Autodesk Inventor part; units mm, degrees
ref_plane "YZ Plane" through (0, 0, 0) normal (1, 0, 0) x (0, 1, 0)
ref_plane "XZ Plane" through (0, 0, 0) normal (0, 1, 0) x (-1, 0, 0)
ref_plane "XY Plane" through (0, 0, 0) normal (0, 0, 1) x (1, 0, 0)
sketch "Skizze1" plane through (0, 0, 0) normal (0, 0, 1) x (1, 0, 0)
  circle A0 centre (0, 0) radius 7.45
  line L0 (-0.9, 9) -> (0.9, 9)
  line L1 (0.9, 9) -> (0.9, -9)
  line L2 (0.9, -9) -> (-0.9, -9)
  line L3 (-0.9, -9) -> (-0.9, 9)
  line L4 (-0.9, 9) -> (0.9, -9) construction
  line L5 (0.9, 9) -> (-0.9, -9) construction
  circle A1 centre (0, 0) radius 2.25
  point P0 (-0.9, -2.0622)
  point P1 (0.9, -2.0622)
  point P2 (0.9, -7.3954)
  point P3 (-0.9, -7.3954)
  dimension "d0" = 14.9
  dimension "d1" = 1.8
  dimension "d2" = 4.5
extrude "Extrusion1" add sketch "Skizze1" along normal blind 3 contours A0 L1 A1 | L1 A1 L3 A0 | L3 A1 A0 picked at (0.4002, 5.6965)
sketch "Skizze2" plane through (0, 0, 3) normal (0, 0, 1) x (1, 0, 0)
  line L0 (0.9, -2.0622) -> (0.9, -7.3954)
  arc A0 (0.9, -7.3954) -> (-0.9, -7.3954) centre (0, 0) ccw
  line L1 (-0.9, -7.3954) -> (-0.9, -2.0622)
  arc A1 (0.9, -2.0622) -> (-0.9, -2.0622) centre (0, 0) ccw
  circle A2 centre (0, 0) radius 10
  line L2 (-0.9, 11.3464) -> (0.9, 11.3464)
  line L3 (0.9, 11.3464) -> (0.9, -11.3464)
  line L4 (0.9, -11.3464) -> (-0.9, -11.3464)
  line L5 (-0.9, -11.3464) -> (-0.9, 11.3464)
  line L6 (-0.9, 11.3464) -> (0.9, -11.3464) construction
  line L7 (0.9, 11.3464) -> (-0.9, -11.3464) construction
  point P0 (-0.9, -9.9594)
  point P1 (-0.9, 2.0622)
  point P2 (-0.9, 7.3954)
  point P3 (0.9, 7.3954)
  point P4 (0.9, 2.0622)
  point P5 (0.9, -9.9594)
  dimension "d5" = 20
  dimension "d6" = 1.8
extrude "Extrusion2" add sketch "Skizze2" along normal blind 0.8 contours A1 L3 A0 L0 | A0 L3 A2 | A1 L5 A0 L3 | A0 L5 A2 L3 | A1 L1 A0 L5 | A0 L5 A2
sketch "Skizze3" plane through (0, 0, 0) normal (0, 0, -1) x (-1, 0, 0)
  line L0 (-0.9, -2.0622) -> (-0.9, -7.3954)
  arc A0 (0.9, -2.0622) -> (-0.9, -2.0622) centre (0, 0) ccw
  line L1 (0.9, -7.3954) -> (0.9, -2.0622)
  arc A1 (0.9, -7.3954) -> (-0.9, -7.3954) centre (0, 0) ccw
  circle A2 centre (0, 0) radius 7.75
  line L2 (0.9, 14.7103) -> (-0.9, 14.7103)
  line L3 (-0.9, 14.7103) -> (-0.9, -14.7103)
  line L4 (-0.9, -14.7103) -> (0.9, -14.7103)
  line L5 (0.9, -14.7103) -> (0.9, 14.7103)
  line L6 (0.9, 14.7103) -> (-0.9, -14.7103) construction
  line L7 (-0.9, 14.7103) -> (0.9, -14.7103) construction
  point P0 (-0.9, -7.6976)
  point P1 (0.9, -7.6976)
  dimension "d9" = 15.5
  dimension "d10" = 1.8
extrude "Extrusion3" add sketch "Skizze3" along normal blind 1.4 contours L0 A1 L3 A0 | L3 A2 A1 | L3 A1 L5 A0 | L3 A2 L5 A1 | L5 A1 L1 A0 | L5 A2 A1
sketch "Skizze4" plane through (0, 0, 3.8) normal (0, 0, 1) x (1, 0, 0)
  circle A0 centre (0, 0) radius 3
extrude "Extrusion4" cut sketch "Skizze4" against normal through all
chamfer "Fase2" distance 0.3 angle 45 1 edges at (0, 7.75, 0)
fillet "Rundung5" radius 6 1 edges at (0, 3, -1.4)
chamfer "Fase3" distance 0.7 angle 45 1 edges at (0, 7.75, -1.4)
fillet "Rundung6" radius 0.5 1 edges at (0, 7.0754, -1.2194)
fillet "Rundung7" radius 0.2 1 edges at (0, 7.75, -0.7)
fillet "Rundung8" radius 0.5 1 edges at (0, 3, 3.8)
properties part number "Buttomplate_BedholePlug"
Geometry: final body of the model. Coordinates: model frame, mm. Give positions to 0.01 mm unless a question says otherwise; leave off trailing zeros. Order: outer loops, then holes, each group sorted by start corner. A loop starts at its lowest first (then second) coordinate and runs counter-clockwise, first axis right, second up. Notation, with made-up numbers: (22.25, 75.25) -> (46.25, 75.25) arc R27 cw to (46.25, 101.25) -> close; hole circle Ø5 at (40, 73.25). An arc over 180 degrees is marked (long way). Write each question's results on one line, items separated by ' | '. Start each with the question number.
1) First-contact query: pin 1 (2 mm diameter, centred on x = 0, y = -6, fed in from -Z); pin 2 (2.5 mm diameter, centred on y = -5.5, z = 0.5, fed in from -X); pin 3 (1 mm diameter, centred on x = 6.5, z = 2, fed in from +Y). Flat tips, straight axial feed; report the tip coordinate or a pass-through.
2) Draft query along Z for faces 1 (the flat face through (4, 0, 3.8)), 2 (the cylindrical face through (-0.315, 7.443, 1.479)), 3 (the conical face through (-0.32, 7.562, -0.119)), 4 (the cylindrical face through (-0.43, 9.99, 3.39)). Return one class per face: pulls with the +Z half, pulls with the -Z half, needs draft (parallel to the pull), parting line crosses it, or undercut.
3) Line query: line 1 (Y direction, x = -2.5, z = 1); line 2 (Z direction, x = 6, y = 0.75); line 3 (X direction, y = -4, z = 0.3). Output: solid intervals per line, ascending. Write a range as from..to.
4) Section A-A (z = 1.95). Return loops of the section in (x, y).
Calculated:
1) pin 1: z = -0.99 | pin 2: x = -6.28 | pin 3: y = 4.42
2) face 1: pulls with the +Z half | face 2: undercut | face 3: undercut | face 4: needs draft
3) line 1: -7.02..-3.21, 3.21..7.02 | line 2: -0.77..3.8 | line 3: -6.29..-2.38, 2.38..6.29
4) outline: (-0.9, -7.4) -> (-0.9, -3.4) arc R3.52 cw (long way) to (0.9, -3.4) -> (0.9, -7.4) arc R7.45 ccw (long way) to start
